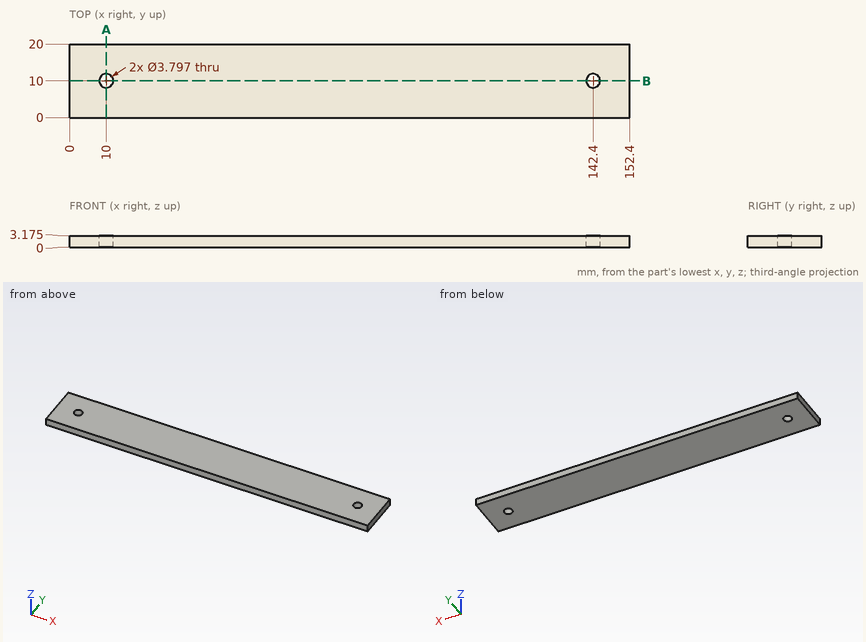
Input: dimensioned drawing with shaded views. Units: mm. Origin: part minimum x, y, z. Coordinates: 2 decimals unless noted, no trailing zeros. Order: outer loops, then holes, each group sorted by start corner. A loop starts at its lowest first (then second) coordinate and runs counter-clockwise, first axis right, second up.
(1) Section query B-B (y = 10). Return the cut outline in (x, z) (1 decimal).
(2) Section query A-A (x = 10). Return the cut outline in (y, z) (1 decimal).
(3) First-contact query: pin 1 (10 mm diameter, centred on x = 30, y = 9.5, fed in from -Z). Flat tip, straight axial feed; report the tip coordinate or a pass-through.
(4) Material intervals for probe 1 along Y at (x, z) = (142.4, 1.7); probe 2 along X at (y, z) = (9.5, 2.95), sorted ascending.
Solution:
1. outline: (0, 0) - (8.1, 0) - (8.1, 3.2) - (0, 3.2) - close; (11.9, 0) - (140.5, 0) - (140.5, 3.2) - (11.9, 3.2) - close; (144.3, 0) - (152.4, 0) - (152.4, 3.2) - (144.3, 3.2) - close
2. outline: (0, 0) - (8.1, 0) - (8.1, 3.2) - (0, 3.2) - close; (11.9, 0) - (20, 0) - (20, 3.2) - (11.9, 3.2) - close
3. pin 1: stops at z = 0
4. probe 1: y = 0 to 8.1, 11.9 to 20
4. probe 2: x = 0 to 8.17, 11.83 to 140.57, 144.23 to 152.4
